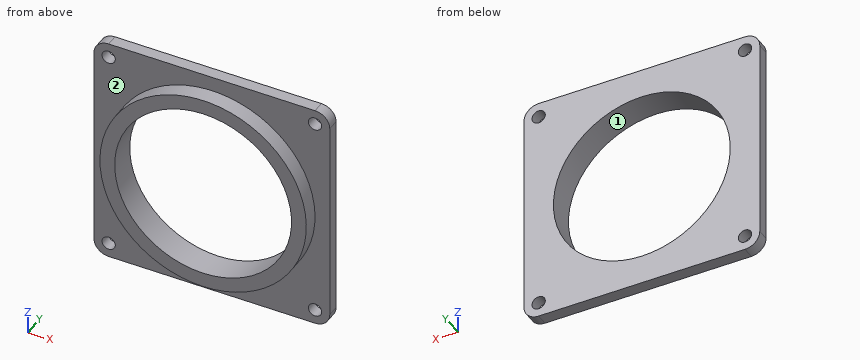
from build123d import *

# Parameters (mm, degrees)
SKETCH1_R           = 35
SKETCH1_R_2         = 30
BOSS_EXTRUDE1_DEPTH = 5.5626
SKETCH2_W           = 80
SKETCH2_H           = 80
SKETCH2_R           = 2.25
SKETCH2_R_2         = 30
BOSS_EXTRUDE3_DEPTH = 4
FILLET1_R           = 5


with BuildPart() as part:
    # Sketch1 → Boss-Extrude1 (new body)
    with BuildSketch(Plane(origin=(0, 0, 0), x_dir=(1, 0, 0), z_dir=(0, 1, 0))):
        with Locations(Location((0, 0, 0), (0, 0, 90))):
            Circle(SKETCH1_R)
        with Locations(Location((0, 0, 0), (0, 0, 90))):
            Circle(SKETCH1_R_2, mode=Mode.SUBTRACT)
    extrude(amount=BOSS_EXTRUDE1_DEPTH)

    # Sketch2 → Boss-Extrude3 (add)
    with BuildSketch(Plane(origin=(0, 5.5626, 0), x_dir=(1, 0, 0), z_dir=(0, 1, 0))):
        Rectangle(SKETCH2_W, SKETCH2_H)
        with Locations(Location((-35, -35, 0), (0, 0, 270))):
            Circle(SKETCH2_R, mode=Mode.SUBTRACT)
        with Locations(Location((-35, 35, 0), (0, 0, 270))):
            Circle(SKETCH2_R, mode=Mode.SUBTRACT)
        with Locations(Location((35, 35, 0), (0, 0, 270))):
            Circle(SKETCH2_R, mode=Mode.SUBTRACT)
        with Locations(Location((35, -35, 0), (0, 0, 270))):
            Circle(SKETCH2_R, mode=Mode.SUBTRACT)
        with Locations(Location((0, 0, 0), (0, 0, 90))):
            Circle(SKETCH2_R_2, mode=Mode.SUBTRACT)
    extrude(amount=BOSS_EXTRUDE3_DEPTH)

    # Fillet1
    fillet1_edges = [part.edges().sort_by_distance(p)[0] for p in [
        (-40, 7.5626, -40),
        (-40, 7.5626, 40),
        (40, 7.5626, 40),
        (40, 7.5626, -40),
    ]]
    fillet(fillet1_edges, radius=FILLET1_R)


solid = part.part
The model under review builds one solid part; all positions refer to its coordinate system, in mm. Face numbers are marked on the shaded views. Coordinates: 2 decimals unless noted, no trailing zeros. Loops run counter-clockwise (first coordinate to the right, second up) from the corner with the lowest first, then second, coordinate; pieces in that order, holes last. Notation, with made-up numbers: (20.25, 63.25) -> (34.25, 63.25) arc R12 cw to (34.25, 86.25) -> close; hole circle Ø3 at (55, 48). An arc over 180 degrees is marked (long way). Use a Markdown table: item, result. Add a question column.
1. Add section A-A on x = 0. Write out the cut boundary in (y, z), plus the area to 3 significant figures.
2. Add section D-D on y = 1.25. Write out the cut boundary in (x, z), plus the area to 3 significant figures.
3. Add section C-C on y = 7. Write out the cut boundary in (x, z).
4. To check wall thickness, follow line 1 (X direction, y = 6.6, z = 35); line 2 (X direction, y = 6, z = 0); line 3 (Y direction, x = 35, z = -21). State the ranges of each line that lie inside material, in increasing order.
5. Draft analysis for pull direction X (two halves, no side actions). For the marked faces 1 and 2, state which applies: pulls with the +X half, pulls with the -X half, needs draft (parallel to the pull), parting line crosses it, or undercut.
6. Add section B-B on z = -18. Write out the cut boundary in (x, y), plus the area to 3 significant figures.
Returned:
| question | item | result |
|---|---|---|
| 1 | outline | (0, -35) -> (5.56, -35) -> (5.56, -40) -> (9.56, -40) -> (9.56, -30) -> (0, -30) -> close; (0, 30) -> (9.56, 30) -> (9.56, 40) -> (5.56, 40) -> (5.56, 35) -> (0, 35) -> close |
| 1 | area | 136 mm² |
| 2 | outline | circle Ø70 at (0, 0); hole circle Ø60 at (0, 0) |
| 2 | area | 1,020 mm² |
| 3 | outline | (-40, -35) arc R5 ccw to (-35, -40) -> (35, -40) arc R5 ccw to (40, -35) -> (40, 35) arc R5 ccw to (35, 40) -> (-35, 40) arc R5 ccw to (-40, 35) -> close; hole circle Ø4.5 at (-35, -35); hole circle Ø4.5 at (-35, 35); hole circle Ø60 at (0, 0); hole circle Ø4.5 at (35, -35); hole circle Ø4.5 at (35, 35) |
| 4 | line 1 | x = -40 to -37.25, -32.75 to 32.75, 37.25 to 40 |
| 4 | line 2 | x = -40 to -30, 30 to 40 |
| 4 | line 3 | y = 5.56 to 9.56 |
| 5 | face 1 | undercut |
| 5 | face 2 | needs draft |
| 6 | outline | (-40, 5.56) -> (-30.02, 5.56) -> (-30.02, 0) -> (-24, 0) -> (-24, 9.56) -> (-40, 9.56) -> close; (24, 0) -> (30.02, 0) -> (30.02, 5.56) -> (40, 5.56) -> (40, 9.56) -> (24, 9.56) -> close |
| 6 | area | 195 mm² |
